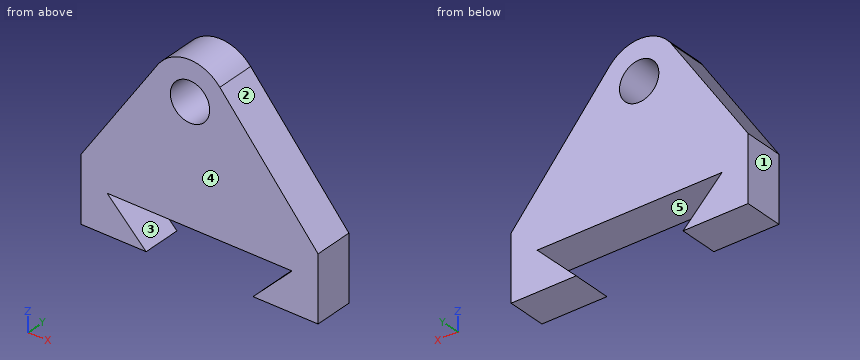
from build123d import *

# Parameters (mm, degrees)
F0_R     = 15.116536
F1_DEPTH = 30


with BuildPart() as f1:
    # F0 (on Front) → F1 (new body)
    with BuildSketch(Plane.XZ):
        with BuildLine():
            ThreePointArc((-24.83029, 58.144077), (-8.806, 12.62944), (30, 41.307905))
            ThreePointArc((30, 41.307905), (28.17257, 51.6184), (22.912913, 60.672781))
            ThreePointArc((22.912913, 60.672781), (-1.586717, 71.265914), (-24.83029, 58.144077))
        make_face()
        with Locations((0, 41.307905)):
            Circle(F0_R, mode=Mode.SUBTRACT)
        with BuildLine():
            ThreePointArc((22.912913, 60.672781), (28.17257, 51.6184), (30, 41.307905))
            ThreePointArc((30, 41.307905), (-8.806, 12.62944), (-24.83029, 58.144077))
            Line((-24.83029, 58.144077), (-83.709534, -28.692095))
            Line((-83.709534, -28.692095), (98.439749, -28.692095))
            Line((98.439749, -28.692095), (22.912913, 60.672781))
        make_face()
        Polygon((98.439749, -78.692095), (98.439749, -28.692095), (-83.709534, -28.692095), (-83.709534, -78.692095), (-33.709534, -78.692095), (-63.709534, -48.692095), (78.439749, -48.692095), (48.439749, -78.692095), align=None)
    extrude(amount=F1_DEPTH)


solid = f1.part
Could you check a few things on this model? Use its own coordinates, in mm. Face numbers are marked on the shaded views. A direction names the side the tool comes from. Give positions to 0.01 mm unless a question says otherwise; leave off trailing zeros. Order: outer loops, then holes, each group sorted by start corner. A loop starts at its lowest first (then second) coordinate and runs counter-clockwise, first axis right, second up. Notation, with made-up numbers: (23, 60) - (35, 60) arc R34 ccw to (35, 99) - close; hole circle Ø1 at (-7, -32). An arc over 180 degrees is marked (long way). One line per question, with ' | ' between items. Start each with the question number.
Item 1: I want a section at C-C on y = -26.5. Write out the boundary of the cut face in (x, z).
Item 2: Thinking about a two-plate mould opening in X: for the marked faces 1, 2 and 3, which applies, pulls with the +X half, pulls with the -X half, needs draft (parallel to the pull), parting line crosses it, or undercut?
Item 3: I want a section at A-A on x = 0. Write out the boundary of the cut face in (y, z), then the cut area to 3 significant figures.
Item 4: I want a section at D-D on z = -6.5. Write out the boundary of the cut face in (x, y), then the cut area to 3 significant figures.
Item 5: For the marked faces 4 and 5, which set-ups out of +Z, -Z, +X, -X, +Y, -Y let a thin tool reach every point of the face, with its end or its side?
Item 6: I'm going to push flat-ended pins straight in: pin 1 Ø12 at (x, y) = (7, -15.5) entering from -Z; pin 2 Ø3 at (y, z) = (-10, 38) entering from -X; pin 3 Ø24 at (x, z) = (0, 41.31) entering from -Y; pin 4 Ø1 at (x, y) = (45, -19) entering from +Z. Where does each tip first touch, or does it pass through?
Item 7: I need wall thicknesses on probe 1 along Z at (x, y) = (0, -7); probe 2 along X at (y, z) = (-18.25, 50); probe 3 along X at (y, z) = (-22, -64.5). Which ranges of each line are inside material? Lowest first, please. Write a range as [from, to].
Item 8: I want a section at B-B on z = -59.5. Write out the boundary of the cut face in (x, y), then the cut area to 3 significant figures.
Verdict:
1) outline: (-83.71, -78.69) - (-33.71, -78.69) - (-63.71, -48.69) - (78.44, -48.69) - (48.44, -78.69) - (98.44, -78.69) - (98.44, -28.69) - (22.91, 60.67) arc R30 ccw to (-24.83, 58.14) - (-83.71, -28.69) - close; hole circle Ø30.23 at (0, 41.31)
2) face 1: pulls with the -X half | face 2: pulls with the +X half | face 3: undercut
3) outline: (-30, -48.69) - (0, -48.69) - (0, 26.19) - (-30, 26.19) - close; (-30, 56.42) - (0, 56.42) - (0, 71.31) - (-30, 71.31) - close | area: 2,690 mm^2
4) outline: (-68.66, -30) - (79.68, -30) - (79.68, 0) - (-68.66, 0) - close | area: 4,450 mm^2
5) face 4: +Z, -Z, +X, -X, -Y | face 5: +Y, -Y
6) pin 1: z = -48.69 | pin 2: x = -39.51 | pin 3: through | pin 4: z = 35.13
7) probe 1: [-48.69, 26.19], [56.42, 71.31] | probe 2: [-30.35, -12.37], [12.37, 31.93] | probe 3: [-83.71, -47.9], [62.63, 98.44]
8) outline: (-83.71, -30) - (-52.9, -30) - (-52.9, 0) - (-83.71, 0) - close; (67.63, -30) - (98.44, -30) - (98.44, 0) - (67.63, 0) - close | area: 1,850 mm^2
